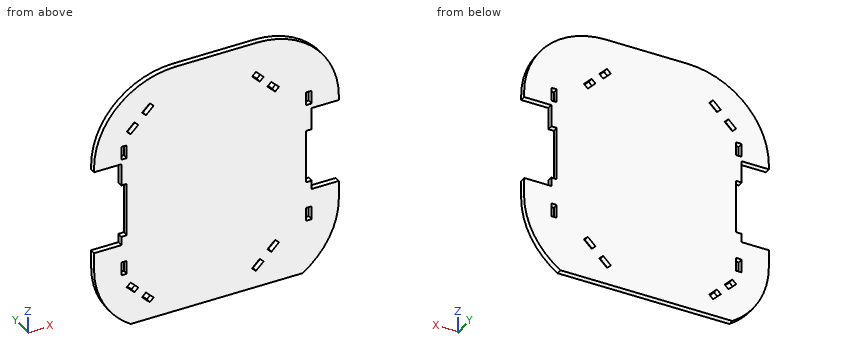
```python
from build123d import *

# Parameters (mm, degrees)
SKETCH1_W            = 228.6
SKETCH1_H            = 241.3
BOSS_EXTRUDE1_DEPTH  = 5.08
SKETCH2_W            = 25.4
SKETCH2_H            = 80
CUT_EXTRUDE1_DEPTH   = 5.08
SKETCH3_W            = 5.08
SKETCH3_H            = 12.7
SKETCH3_H_2          = 50.8
CUT_EXTRUDE2_DEPTH   = 5.08
CUT_EXTRUDE3_REACH   = 7.08
CUT_EXTRUDE4_DEPTH   = 5.08
MIRROR4_COPY_1_DEPTH = 5.08


with BuildPart() as part:
    # Sketch1 → Boss-Extrude1 (new body)
    with BuildSketch(Plane(origin=(0, 0, 0), x_dir=(1, 0, 0), z_dir=(0, 1, 0))):
        with Locations((114.3, 120.65)):
            Rectangle(SKETCH1_W, SKETCH1_H)
    extrude(amount=BOSS_EXTRUDE1_DEPTH)

    # Sketch2 → Cut-Extrude1 (cut)
    with BuildSketch(Plane(origin=(0, 5.08, 0), x_dir=(1, 0, 0), z_dir=(0, 1, 0))):
        with Locations((12.7, 120.65)):
            Rectangle(SKETCH2_W, SKETCH2_H)
    cut_extrude1 = extrude(amount=-CUT_EXTRUDE1_DEPTH, mode=Mode.SUBTRACT)

    # Mirror1: Cut-Extrude1 across plane
    add(cut_extrude1.mirror(Plane.ZY.offset(-114.3)), mode=Mode.SUBTRACT)

    # Sketch3 → Cut-Extrude2 (cut)
    with BuildSketch(Plane.XZ):
        with Locations((27.94, -184.15)):
            Rectangle(SKETCH3_W, SKETCH3_H)
        with Locations((27.94, -127)):
            Rectangle(SKETCH3_W, SKETCH3_H_2)
        with Locations((27.94, -69.85)):
            Rectangle(SKETCH3_W, SKETCH3_H)
    cut_extrude2 = extrude(amount=-CUT_EXTRUDE2_DEPTH, mode=Mode.SUBTRACT)

    # Mirror2: Cut-Extrude2 across plane
    add(cut_extrude2.mirror(Plane.ZY.offset(-114.3)), mode=Mode.SUBTRACT)

    # Sketch4 → Cut-Extrude3 (cut, up to next)
    with BuildSketch(Plane.XZ, mode=Mode.PRIVATE) as cut_extrude3_sk1:
        Polygon((55.639202938, -221.813411753), (48.454998041, -214.629206856), (44.862895593, -218.221309304), (52.047100489, -225.405514201), align=None)
    cut_extrude3_tool1 = extrude(cut_extrude3_sk1.sketch, amount=-CUT_EXTRUDE3_REACH, mode=Mode.PRIVATE) & part.part
    add(cut_extrude3_tool1.solids().sort_by_distance((50.251049, 0, -220.017361))[0], mode=Mode.SUBTRACT)
    # Sketch4 → Cut-Extrude3 (cut, up to next)
    with BuildSketch(Plane.XZ, mode=Mode.PRIVATE) as cut_extrude3_sk2:
        Polygon((41.270793144, -207.445001959), (34.086588247, -200.260797062), (30.494485799, -203.852899511), (37.678690696, -211.037104407), align=None)
    cut_extrude3_tool2 = extrude(cut_extrude3_sk2.sketch, amount=-CUT_EXTRUDE3_REACH, mode=Mode.PRIVATE) & part.part
    add(cut_extrude3_tool2.solids().sort_by_distance((35.882639, 0, -205.648951))[0], mode=Mode.SUBTRACT)
    # Sketch4 → Cut-Extrude3 (cut, up to next)
    with BuildSketch(Plane.XZ, mode=Mode.PRIVATE) as cut_extrude3_sk3:
        Polygon((34.086588247, -53.739202938), (41.270793144, -46.554998041), (37.678690696, -42.962895593), (30.494485799, -50.147100489), align=None)
    cut_extrude3_tool3 = extrude(cut_extrude3_sk3.sketch, amount=-CUT_EXTRUDE3_REACH, mode=Mode.PRIVATE) & part.part
    add(cut_extrude3_tool3.solids().sort_by_distance((35.882639, 0, -48.351049))[0], mode=Mode.SUBTRACT)
    # Sketch4 → Cut-Extrude3 (cut, up to next)
    with BuildSketch(Plane.XZ, mode=Mode.PRIVATE) as cut_extrude3_sk4:
        Polygon((48.454998041, -39.370793144), (55.639202938, -32.186588247), (52.047100489, -28.594485799), (44.862895593, -35.778690696), align=None)
    cut_extrude3_tool4 = extrude(cut_extrude3_sk4.sketch, amount=-CUT_EXTRUDE3_REACH, mode=Mode.PRIVATE) & part.part
    add(cut_extrude3_tool4.solids().sort_by_distance((50.251049, 0, -33.982639))[0], mode=Mode.SUBTRACT)
    # Sketch4 → Cut-Extrude3 (cut, up to next)
    with BuildSketch(Plane.XZ, mode=Mode.PRIVATE) as cut_extrude3_sk5:
        Polygon((147.560797062, -32.186588247), (154.745001959, -39.370793144), (158.337104407, -35.778690696), (151.152899511, -28.594485799), align=None)
    cut_extrude3_tool5 = extrude(cut_extrude3_sk5.sketch, amount=-CUT_EXTRUDE3_REACH, mode=Mode.PRIVATE) & part.part
    add(cut_extrude3_tool5.solids().sort_by_distance((152.948951, 0, -33.982639))[0], mode=Mode.SUBTRACT)
    # Sketch4 → Cut-Extrude3 (cut, up to next)
    with BuildSketch(Plane.XZ, mode=Mode.PRIVATE) as cut_extrude3_sk6:
        Polygon((161.929206856, -46.554998041), (169.113411753, -53.739202938), (172.705514201, -50.147100489), (165.521309304, -42.962895593), align=None)
    cut_extrude3_tool6 = extrude(cut_extrude3_sk6.sketch, amount=-CUT_EXTRUDE3_REACH, mode=Mode.PRIVATE) & part.part
    add(cut_extrude3_tool6.solids().sort_by_distance((167.317361, 0, -48.351049))[0], mode=Mode.SUBTRACT)
    # Sketch4 → Cut-Extrude3 (cut, up to next)
    with BuildSketch(Plane.XZ, mode=Mode.PRIVATE) as cut_extrude3_sk7:
        Polygon((154.745001959, -214.629206856), (147.560797062, -221.813411753), (151.152899511, -225.405514201), (158.337104407, -218.221309304), align=None)
    cut_extrude3_tool7 = extrude(cut_extrude3_sk7.sketch, amount=-CUT_EXTRUDE3_REACH, mode=Mode.PRIVATE) & part.part
    add(cut_extrude3_tool7.solids().sort_by_distance((152.948951, 0, -220.017361))[0], mode=Mode.SUBTRACT)
    # Sketch4 → Cut-Extrude3 (cut, up to next)
    with BuildSketch(Plane.XZ, mode=Mode.PRIVATE) as cut_extrude3_sk8:
        Polygon((169.113411753, -200.260797062), (161.929206856, -207.445001959), (165.521309304, -211.037104407), (172.705514201, -203.852899511), align=None)
    cut_extrude3_tool8 = extrude(cut_extrude3_sk8.sketch, amount=-CUT_EXTRUDE3_REACH, mode=Mode.PRIVATE) & part.part
    add(cut_extrude3_tool8.solids().sort_by_distance((167.317361, 0, -205.648951))[0], mode=Mode.SUBTRACT)

    # Sketch5 → Cut-Extrude4 (cut)
    with BuildSketch(Plane.XZ):
        with BuildLine():
            Line((0, -76.2), (0, 0))
            Line((0, 0), (76.2, 0))
            ThreePointArc((76.2, 0), (22.318463274, -22.318463274), (0, -76.2))
        make_face()
    cut_extrude4 = extrude(amount=-CUT_EXTRUDE4_DEPTH, mode=Mode.SUBTRACT)

    # Mirror3: Cut-Extrude4 across plane
    add(cut_extrude4.mirror(Plane.ZY.offset(-114.3)), mode=Mode.SUBTRACT)

    # Mirror4: Cut-Extrude4 across plane
    add(cut_extrude4.mirror(Plane.XY.offset(-127)), mode=Mode.SUBTRACT)

    # Mirror4 copy 1 sketch → Mirror4 copy 1 (cut)
    with BuildSketch(Plane(origin=(228.6, 0, -254), x_dir=(-1, 0, 0), z_dir=(0, -1, 0))):
        with BuildLine():
            Line((0, -76.2), (0, 0))
            Line((0, 0), (76.2, 0))
            ThreePointArc((76.2, 0), (22.318463274, -22.318463274), (0, -76.2))
        make_face()
    extrude(amount=-MIRROR4_COPY_1_DEPTH, mode=Mode.SUBTRACT)


solid = part.part
```
Could you check a few things on this model? Use its own coordinates, in mm. Coordinates: 2 decimals unless noted, no trailing zeros. Loops run counter-clockwise (first coordinate to the right, second up) from the corner with the lowest first, then second, coordinate; pieces in that order, holes last.
1) Will these pins go through, and if not, where does the flat tip stop? pin 1 Ø2.5 at (y, z) = (2, -86) entering from -X; pin 2 Ø2.5 at (x, y) = (199.5, 3.5) entering from -Z; pin 3 Ø2.5 at (y, z) = (1.5, -184.5) entering from -X; pin 4 Ø12 at (x, z) = (141.5, -165.5) entering from -Y.
Reported:
pin 1: stops at x = 25.4
pin 2: stops at z = -238.66
pin 3: stops at x = 0.2
pin 4: stops at y = 0
2) Imagine slicing it at D-D (z = -18). List the corners of the cut face in (x, y) for me.
Reported:
outline: (27.01, 0) - (201.59, 0) - (201.59, 5.08) - (27.01, 5.08) - close
3) Imagine slicing it at B-B (y = 2.6). State how many separate pieces and enclosed holes the cut face has, and give its area (3 significant figures).
Reported:
separate pieces: 1
enclosed holes: 12
area: 46,100 mm2
4) Please list where these lines run through material, in increasing order: line 1 along X through (y, z) = (2.65, -218); line 2 along X through (y, z) = (3.75, -206); line 3 along X through (y, z) = (1.45, -94).
Reported:
line 1: x = 11.47 to 45.08, 51.83 to 151.37, 158.12 to 217.13
line 2: x = 5.41 to 32.64, 39.83 to 163.37, 170.56 to 223.19
line 3: x = 25.4 to 203.2
5) Imagine slicing it at A-A (x = 212.5). List the corners of the cut face in (y, z) for me, and give its area (3 significant figures).
Reported:
outline: (0, -224.64) - (5.08, -224.64) - (5.08, -160.65) - (0, -160.65) - close; (0, -80.65) - (5.08, -80.65) - (5.08, -29.36) - (0, -29.36) - close
area: 586 mm2
6) Imagine slicing it at C-C (z = -94.5). List the corners of the cut face in (x, y) for me, and give its area (3 significant figures).
Reported:
outline: (25.4, 0) - (203.2, 0) - (203.2, 5.08) - (25.4, 5.08) - close
area: 903 mm2
